```python
from build123d import *

# Parameters (mm, degrees)
BOSS_EXTRU_1_DEPTH = 2
ESQUISSE4_W        = 2
ESQUISSE4_H        = 33
BOSS_EXTRU_2_DEPTH = 7
ESQUISSE6_W        = 60
ESQUISSE6_H        = 33
BOSS_EXTRU_3_DEPTH = 2
ESQUISSE7_W        = 2
ESQUISSE7_H        = 31
BOSS_EXTRU_4_DEPTH = 7
ESQUISSE8_R        = 5
BOSS_EXTRU_5_DEPTH = 5
ESQUISSE9_R        = 2.5
BOSS_EXTRU_6_DEPTH = 3


with BuildPart() as part:
    # Esquisse1 → Boss.-Extru.1 (new body)
    with BuildSketch(Plane(origin=(0, 0, 0), x_dir=(1, 0, 0), z_dir=(0, 1, 0))):
        Polygon((8.388206388, 24.250614251), (26.388206388, 24.250614251), (26.388206388, -35.749385749), (8.388206388, -35.749385749), (8.388206388, -42.749385749), (-23.611793612, -42.749385749), (-23.611793612, -35.749385749), (-23.611793612, 24.250614251), (-23.611793612, 31.250614251), (8.388206388, 31.250614251), align=None)
    extrude(amount=BOSS_EXTRU_1_DEPTH)

    # Esquisse4 → Boss.-Extru.2 (add)
    with BuildSketch(Plane.XY.offset(42.749385749)):
        with Locations((-22.611793612, 16.5)):
            Rectangle(ESQUISSE4_W, ESQUISSE4_H)
    extrude(amount=-BOSS_EXTRU_2_DEPTH)

    # Esquisse6 → Boss.-Extru.3 (add)
    with BuildSketch(Plane(origin=(26.388206388, 0, 0), x_dir=(0, 0, -1), z_dir=(1, 0, 0))):
        with Locations((-5.749385749, 16.5)):
            Rectangle(ESQUISSE6_W, ESQUISSE6_H)
    extrude(amount=-BOSS_EXTRU_3_DEPTH)

    # Esquisse7 → Boss.-Extru.4 (add)
    with BuildSketch(Plane(origin=(0, 0, -31.250614251), x_dir=(-1, 0, 0), z_dir=(0, 0, -1))):
        with Locations((22.611793612, 15.5)):
            Rectangle(ESQUISSE7_W, ESQUISSE7_H)
    extrude(amount=-BOSS_EXTRU_4_DEPTH)

    # Esquisse8 → Boss.-Extru.5 (add)
    with BuildSketch(Plane(origin=(26.388206388, 0, 0), x_dir=(0, 0, -1), z_dir=(1, 0, 0))):
        with Locations((14.127664827, 16.462750596)):
            Circle(ESQUISSE8_R)
    extrude(amount=BOSS_EXTRU_5_DEPTH)

    # Esquisse9 → Boss.-Extru.6 (add)
    with BuildSketch(Plane(origin=(31.388206388, 0, 0), x_dir=(0, 0, -1), z_dir=(1, 0, 0))):
        with Locations((14.127664827, 16.462750596)):
            Circle(ESQUISSE9_R)
    extrude(amount=BOSS_EXTRU_6_DEPTH)


solid = part.part
```
Geometry check sheet. Reference: the model listing, model coordinates, mm. A direction names the side the tool comes from. Give positions to 0.01 mm unless a question says otherwise; leave off trailing zeros. Order: outer loops, then holes, each group sorted by start corner. A loop starts at its lowest first (then second) coordinate and runs counter-clockwise, first axis right, second up.
1. Gauge pin test, flat ends, axial feed: pin 1 Ø0.6 at (y, z) = (1, 38.5) entering from +X; pin 2 Ø6 at (x, y) = (23, 17) entering from +Z; pin 3 Ø7.5 at (y, z) = (13.5, 38) entering from +X. Record the tip position at first contact, or that the pin passes through.
2. Section check C-C, the plane x = -6. Enter the section's corners in (y, z), and give its area (3 significant figures).
3. Section check A-A, the plane y = 5. Enter the section's corners in (x, z), and give its area (3 significant figures).
4. Access from +Z, -Z, +X, -X, +Y, -Y to the whole of each face (thin tool, end or side, straight path). Record for faces 4 (the face through (-23, 31, -28)), 5 (the face through (25, 10, -24.251)), 6 (the face through (8.388, 1, 39)), 7 (the face through (-21.612, 17, 39)), 8 (the face through (32.87, 16.57, -11.63)).
5. Release check for a two-part mould opening along Z. For faces 1 (the face through (25, 12, 35.749)), 2 (the face through (-21.612, 16, -28)), 3 (the face through (-23, 17, -24.251)) record: pulls with the +Z half, pulls with the -Z half, needs draft (parallel to the pull), parting line crosses it, or undercut.
6. Section check B-B, the plane z = 10. Enter the section's corners in (x, y).
7. Section check D-D, the plane y = 12.5. Enter the section's corners in (x, z).
8. Thickness scan on L1, parallel to Y at x = -13, z = -4.5; L2, parallel to Z at x = 25, y = 14; L3, parallel to X at y = 30, z = 39. Record the ranges inside material, lowest first.
Values follow:
1. pin 1: stops at x = 8.39
1. pin 2: stops at z = 35.75
1. pin 3: stops at x = 26.39
2. outline: (0, -31.25) - (2, -31.25) - (2, 42.75) - (0, 42.75) - close
2. area: 148 mm2
3. outline: (-23.61, -31.25) - (-21.61, -31.25) - (-21.61, -24.25) - (-23.61, -24.25) - close; (-23.61, 35.75) - (-21.61, 35.75) - (-21.61, 42.75) - (-23.61, 42.75) - close; (24.39, -24.25) - (26.39, -24.25) - (26.39, 35.75) - (24.39, 35.75) - close
3. area: 148 mm2
4. face 4: -Z, +X, -X, +Y
4. face 5: -Z, +X, +Y, -Y
4. face 6: +Z, +X, +Y, -Y
4. face 7: +Z, -Z, +X, +Y
4. face 8: +X
5. face 1: pulls with the +Z half
5. face 2: needs draft
5. face 3: undercut
6. outline: (-23.61, 0) - (26.39, 0) - (26.39, 33) - (24.39, 33) - (24.39, 2) - (-23.61, 2) - close
7. outline: (-23.61, -31.25) - (-21.61, -31.25) - (-21.61, -24.25) - (-23.61, -24.25) - close; (-23.61, 35.75) - (-21.61, 35.75) - (-21.61, 42.75) - (-23.61, 42.75) - close; (24.39, -24.25) - (26.39, -24.25) - (26.39, -17.18) - (31.39, -17.18) - (31.39, -11.08) - (26.39, -11.08) - (26.39, 35.75) - (24.39, 35.75) - close
8. L1: y = 0 to 2
8. L2: z = -24.25 to 35.75
8. L3: x = -23.61 to -21.61
